from build123d import *

# Parameters (mm, degrees)
SKETCH_1_R               = 5
EXTRUDE_1_DEPTH          = 5
SKETCH_3_W               = 200
SKETCH_3_H               = 180
EXTRUDE_2_DEPTH          = 8
SKETCH_4_W               = 140
SKETCH_4_H               = 125
CUT_EXTRUDE_1_DEPTH      = 1
CUT_EXTRUDE_2_DEPTH      = 150.629542538
CUT_EXTRUDE_2_DEPTH_BACK = 150.629542538
SKETCH_6_W               = 20
SKETCH_6_H               = 3
CUT_EXTRUDE_3_DEPTH      = 5


with BuildPart() as part:
    # 草图1 → 凸台-拉伸1 (new, symmetric)
    with BuildSketch(Plane.XY):
        with BuildLine():
            Line((-100, -100), (100, -100))
            ThreePointArc((100, -100), (107.071067812, -97.071067812), (110, -90))
            Line((110, -90), (110, 90))
            ThreePointArc((110, 90), (107.071067812, 97.071067812), (100, 100))
            Line((100, 100), (-100, 100))
            ThreePointArc((-100, 100), (-107.071067812, 97.071067812), (-110, 90))
            Line((-110, 90), (-110, -90))
            ThreePointArc((-110, -90), (-107.071067812, -97.071067812), (-100, -100))
        make_face()
        with Locations((-90, 0)):
            Circle(SKETCH_1_R, mode=Mode.SUBTRACT)
        with Locations((90, 0)):
            Circle(SKETCH_1_R, mode=Mode.SUBTRACT)
        with Locations((-90, 40)):
            Circle(SKETCH_1_R, mode=Mode.SUBTRACT)
        with Locations((-90, -40)):
            Circle(SKETCH_1_R, mode=Mode.SUBTRACT)
        with Locations(Location((90, -40, 0), (0, 0, 180))):
            Circle(SKETCH_1_R, mode=Mode.SUBTRACT)
        with Locations(Location((90, 40, 0), (0, 0, 180))):
            Circle(SKETCH_1_R, mode=Mode.SUBTRACT)
        with Locations((-90, -80)):
            Circle(SKETCH_1_R, mode=Mode.SUBTRACT)
        with Locations((-90, 80)):
            Circle(SKETCH_1_R, mode=Mode.SUBTRACT)
        with Locations(Location((90, -80, 0), (0, 0, 180))):
            Circle(SKETCH_1_R, mode=Mode.SUBTRACT)
        with Locations(Location((90, 80, 0), (0, 0, 180))):
            Circle(SKETCH_1_R, mode=Mode.SUBTRACT)
        with Locations((0, 80)):
            Circle(SKETCH_1_R, mode=Mode.SUBTRACT)
        with Locations((-45, 80)):
            Circle(SKETCH_1_R, mode=Mode.SUBTRACT)
        with Locations((45, 80)):
            Circle(SKETCH_1_R, mode=Mode.SUBTRACT)
        with Locations(Location((45, -80, 0), (0, 0, 180))):
            Circle(SKETCH_1_R, mode=Mode.SUBTRACT)
        with Locations(Location((0, -80, 0), (0, 0, 180))):
            Circle(SKETCH_1_R, mode=Mode.SUBTRACT)
        with Locations(Location((-45, -80, 0), (0, 0, 180))):
            Circle(SKETCH_1_R, mode=Mode.SUBTRACT)
    extrude(amount=EXTRUDE_1_DEPTH, both=True)

    # 草图3 → 凸台-拉伸2 (add)
    with BuildSketch(Plane(origin=(0, 0, -5), x_dir=(-1, 0, 0), z_dir=(0, 0, -1))):
        with BuildLine():
            Line((110, 90), (110, -90))
            ThreePointArc((110, -90), (107.071067812, -97.071067812), (100, -100))
            Line((100, -100), (-100, -100))
            ThreePointArc((-100, -100), (-107.071067812, -97.071067812), (-110, -90))
            Line((-110, -90), (-110, 90))
            ThreePointArc((-110, 90), (-107.071067812, 97.071067812), (-100, 100))
            Line((-100, 100), (100, 100))
            ThreePointArc((100, 100), (107.071067812, 97.071067812), (110, 90))
        make_face()
        Rectangle(SKETCH_3_W, SKETCH_3_H, mode=Mode.SUBTRACT)
    extrude(amount=EXTRUDE_2_DEPTH)

    # 草图4 → 切除-拉伸1 (cut)
    with BuildSketch(Plane.XY.offset(5)):
        Rectangle(SKETCH_4_W, SKETCH_4_H)
    extrude(amount=-CUT_EXTRUDE_1_DEPTH, mode=Mode.SUBTRACT)

    # 草图5 → 切除-拉伸2 (cut, two sides: drawn at the far end of the back side and taken through both)
    with BuildSketch(Plane.XY.offset(4).offset(-CUT_EXTRUDE_2_DEPTH_BACK)):
        Polygon((0, -62.5), (10, -62.5), (10, -59.5), (-10, -59.5), (-10, -62.5), align=None)
    extrude(amount=CUT_EXTRUDE_2_DEPTH + CUT_EXTRUDE_2_DEPTH_BACK, mode=Mode.SUBTRACT)

    # 草图6 → 切除-拉伸3 (cut)
    with BuildSketch(Plane.XZ.offset(100)):
        with Locations((0, -11.5)):
            Rectangle(SKETCH_6_W, SKETCH_6_H)
    extrude(amount=-CUT_EXTRUDE_3_DEPTH, mode=Mode.SUBTRACT)


solid = part.part
Work out the finished part from the listing and answer in its coordinate system (mm). A direction names the side the tool comes from. Give positions to 0.01 mm unless a question says otherwise; leave off trailing zeros. Loops run counter-clockwise (first coordinate to the right, second up) from the corner with the lowest first, then second, coordinate; pieces in that order, holes last. Notation, with made-up numbers: (69.5, 52.25) - (102.5, 52.25) arc R37 cw to (102.5, 88.25) - close; hole circle Ø5 at (89, 39.5). An arc over 180 degrees is marked (long way). Answer in a Markdown table with one row per item. Add a question column.
Q1. A tool of negligible diameter and unlimited length cuts with its end or side. For faces 1 (the flat face through (0, -59.5, -1)), 2 (the flat face through (0, -62.5, 2)), 3 (the flat face through (0, -98, -10)), 4 (the flat face through (-2, 68, 5)), 5 (the flat face through (1, 90, -9)), from which of +Z, -Z, +X, -X, +Y, -Y can it reach the whole face along a straight path? Write none if from no direction.
Q2. Each of these flat-tipped pins is pushed along its axis until it touches: P1, Ø6, axis at x = 29, y = -55.5, coming from the -Z side; P2, Ø8, axis at x = 90, y = 40, coming from the -Z side; P3, Ø0.9, axis at x = -3.5, z = -12, coming from the -Y side; P4, Ø2.5, axis at y = -97.5, z = -12, coming from the -X side. Where does it stop, or does it pass through?
Q3. Consider line 1 along Y through (x, z) = (-90, -3); line 2 along Y through (x, z) = (-46, -8.25); line 3 along X through (y, z) = (-89, -6.25). Determine where each line is inside the solid, lowest interval first.
Q4. The part is cut by section C-C (z = 0). State how many separate pieces and enclosed holes the cut face has, and give its area (3 significant figures).
Q5. The part is cut by section D-D (y = 80). Determine the outline of the cut face in (x, z).
Q6. The part is cut by section B-B (y = -40). Determine the outline of the cut face in (x, z).
Q7. The part is cut by section A-A (x = 45). Determine the outline of the cut face in (y, z), and give its area (4 significant figures).
Q8. Determine the mould class of faces 6 (the flat face through (-1, 1, 4)), 7 (the flat face through (-1, -100, -4)), 8 (the cylindrical face through (-106.99, 97.15, -3.87)) for opening direction Y: released by +Y, released by -Y, zero draft, split by the parting line, or undercut.
Solution:
| question | item | result |
|---|---|---|
| 1 | face 1 | +Z, -Z |
| 1 | face 2 | +Z |
| 1 | face 3 | -Z, -Y |
| 1 | face 4 | +Z, +X, -X, +Y, -Y |
| 1 | face 5 | -Z |
| 2 | P1 | stops at z = -5 |
| 2 | P2 | passes through |
| 2 | P3 | stops at y = -95 |
| 2 | P4 | stops at x = -107.81 |
| 3 | line 1 | y = -100 to -85, -75 to -45, -35 to -5, 5 to 35, 45 to 75, 85 to 100 |
| 3 | line 2 | y = -100 to -90, 90 to 100 |
| 3 | line 3 | x = -110 to -100, 100 to 110 |
| 4 | separate pieces | 1 |
| 4 | enclosed holes | 17 |
| 4 | area | 42,600 mm² |
| 5 | outline | (-110, -13) - (-100, -13) - (-100, -5) - (-95, -5) - (-95, 5) - (-110, 5) - close; (-85, -5) - (-50, -5) - (-50, 5) - (-85, 5) - close; (-40, -5) - (-5, -5) - (-5, 5) - (-40, 5) - close; (5, -5) - (40, -5) - (40, 5) - (5, 5) - close; (50, -5) - (85, -5) - (85, 5) - (50, 5) - close; (95, -5) - (100, -5) - (100, -13) - (110, -13) - (110, 5) - (95, 5) - close |
| 6 | outline | (-110, -13) - (-100, -13) - (-100, -5) - (-95, -5) - (-95, 5) - (-110, 5) - close; (-85, -5) - (85, -5) - (85, 5) - (70, 5) - (70, 4) - (-70, 4) - (-70, 5) - (-85, 5) - close; (95, -5) - (100, -5) - (100, -13) - (110, -13) - (110, 5) - (95, 5) - close |
| 7 | outline | (-100, -13) - (-90, -13) - (-90, -5) - (-85, -5) - (-85, 5) - (-100, 5) - close; (-75, -5) - (75, -5) - (75, 5) - (62.5, 5) - (62.5, 4) - (-62.5, 4) - (-62.5, 5) - (-75, 5) - close; (85, -5) - (90, -5) - (90, -13) - (100, -13) - (100, 5) - (85, 5) - close |
| 7 | area | 1,835 mm² |
| 8 | face 6 | undercut |
| 8 | face 7 | released by -Y |
| 8 | face 8 | released by +Y |
